Check sheet for the modelled part. Datum: model origin and axes. Units: mm. A direction names the side the tool comes from. Round coordinates to 2 decimals unless told otherwise and drop trailing zeros. Order: outer loops, then holes, each group sorted by start corner. A loop starts at its lowest first (then second) coordinate and runs counter-clockwise, first axis right, second up. Notation, with made-up numbers: M -24.75,82.5 L 3.25,82.5 A33 cw 3.25,112.5 Z; hole C -33,-22.5 d11. An arc over 180 degrees is marked long. One line per item, written item: value. Start each with the question number.
(1) Release check for a two-part mould opening along X. For faces 4 (the face through (0, 21, 5)), 5 (the face through (-17, 10, 5)), 6 (the face through (0, 18.6, 3)) record: released by +X, released by -X, zero draft, split by the parting line, or undercut.
(2) Access from +Z, -Z, +X, -X, +Y, -Y to the whole of each face (thin tool, end or side, straight path). Record for faces 1 (the face through (0, 1.4, 6)), 2 (the face through (16, 10, 5)), 3 (the face through (-1, 20, 10)).
(3) Depth check by flat-ended pin: pin 1 Ø6 at (x, z) = (8.5, 4.5) entering from -Y; pin 2 Ø5.5 at (x, y) = (10.34, 10.78) entering from +Z; pin 3 Ø2 at (x, y) = (-9.66, 10.78) entering from -Z. Enter the tip coordinate at first touch or a pass-through.
(4) Thickness scan on L1, parallel to X at y = 4.75, z = 8.5; L2, parallel to Y at x = 7, z = 7.5; L3, parallel to Z at x = 12.5, y = 7.5. Record the ranges inside material, lowest first.
(5) Cross-section at D-D, the plane y = 11.75. Enter the section's corners in (x, z), and give its area (3 significant figures).
(6) Cross-section at C-C, the plane z = 7.75. Enter the section's corners in (x, y).
from build123d import *

# Parameters (mm, degrees)
SKETCH_W        = 34
SKETCH_H        = 21
PAD_DEPTH       = 10
SKETCH001_W     = 31.2
SKETCH001_H     = 18.2
POCKET_DEPTH    = 8
SKETCH002_W     = 31.192015
SKETCH002_H     = 1
PAD001_DEPTH    = 3
SKETCH003_W     = 31.192015
SKETCH003_H     = 1
PAD002_DEPTH    = 3
SKETCH004_W     = 9
SKETCH004_H     = 5
POCKET001_DEPTH = 5
SKETCH005_W     = 31.192015
SKETCH005_H     = 0.5
PAD003_DEPTH    = 0.3
SKETCH006_W     = 31.116258
SKETCH006_H     = 0.5
PAD004_DEPTH    = 0.3
SKETCH007_R     = 1.75
POCKET002_DEPTH = 5


with BuildPart() as part:
    # Sketch → Pad (new body)
    with BuildSketch(Plane.XY):
        with Locations((0, 10.5)):
            Rectangle(SKETCH_W, SKETCH_H)
    extrude(amount=PAD_DEPTH)

    # Sketch001 (on Face6 of Pad) → Pocket (cut)
    with BuildSketch(Plane.XY.offset(10)):
        with Locations((0, 10.5)):
            Rectangle(SKETCH001_W, SKETCH001_H)
    extrude(amount=-POCKET_DEPTH, mode=Mode.SUBTRACT)

    # Sketch002 (on Face11 of Pocket) → Pad001 (join)
    with BuildSketch(Plane.XY.offset(2)):
        with Locations((-0.0039925, 19.1)):
            Rectangle(SKETCH002_W, SKETCH002_H)
    extrude(amount=PAD001_DEPTH)

    # Sketch003 (on Face13 of Pad001) → Pad002 (join)
    with BuildSketch(Plane.XY.offset(2)):
        with Locations((-0.0797495, 1.931894)):
            Rectangle(SKETCH003_W, SKETCH003_H)
    extrude(amount=PAD002_DEPTH)

    # Sketch004 (on Face3 of Pad002) → Pocket001 (cut)
    with BuildSketch(Plane.YZ.offset(17)):
        with Locations((10.5, 7.5)):
            Rectangle(SKETCH004_W, SKETCH004_H)
    extrude(amount=-POCKET001_DEPTH, mode=Mode.SUBTRACT)

    # Sketch005 (on Face11 of Pocket001) → Pad003 (join)
    with BuildSketch(Plane.XZ.offset(-19.6)):
        with Locations((-0.0039925, 6.85)):
            Rectangle(SKETCH005_W, SKETCH005_H)
    extrude(amount=PAD003_DEPTH)

    # Sketch006 (on Face13 of Pad003) → Pad004 (join)
    with BuildSketch(Plane(origin=(0, 1.4, 0), x_dir=(-1, 0, 0), z_dir=(0, 1, 0))):
        with Locations((0.041871, 6.85)):
            Rectangle(SKETCH006_W, SKETCH006_H)
    extrude(amount=PAD004_DEPTH)

    # Sketch007 (on Face14 of Pad004) → Pocket002 (cut)
    with BuildSketch(Plane.XY.offset(2)):
        with Locations((-9.6637815806, 10.781894)):
            Circle(SKETCH007_R)
        with Locations((10.3362184194, 10.781894)):
            Circle(SKETCH007_R)
    extrude(amount=-POCKET002_DEPTH, mode=Mode.SUBTRACT)


solid = part.part
Values found:
1. face 4: zero draft
1. face 5: released by -X
1. face 6: undercut
2. face 1: none
2. face 2: +Z, +X
2. face 3: +Z, +X, -X, +Y, -Y
3. pin 1: y = 0
3. pin 2: z = 2
3. pin 3: through
4. L1: -17 to -15.6, 15.6 to 17
4. L2: 0 to 1.4, 19.6 to 21
4. L3: 0 to 2
5. outline: M -17,0 L -11.12,0 L -11.12,2 L -15.6,2 L -15.6,10 L -17,10 Z; M -8.21,0 L 8.88,0 L 8.88,2 L -8.21,2 Z; M 11.79,0 L 17,0 L 17,5 L 15.6,5 L 15.6,2 L 11.79,2 Z
5. area: 71.7 mm^2
6. outline: M -17,0 L 17,0 L 17,6 L 15.6,6 L 15.6,1.4 L -15.6,1.4 L -15.6,19.6 L 15.6,19.6 L 15.6,15 L 17,15 L 17,21 L -17,21 Z
